The figure shows three views and two pictorial views of one solid part (mm, origin at its lowest corner). Answer the questions. Round coordinates to 2 decimals unless told otherwise and drop trailing zeros. Order: outer loops, then holes, each group sorted by start corner. A loop starts at its lowest first (then second) coordinate and runs counter-clockwise, first axis right, second up. Notation, with made-up numbers: (73, -40) - (95, -40) arc R16 cw to (95, -22) - close; hole circle Ø2 at (19.25, 76.5). An arc over 180 degrees is marked (long way). One line per question, with ' | ' between items. Start each with the question number.
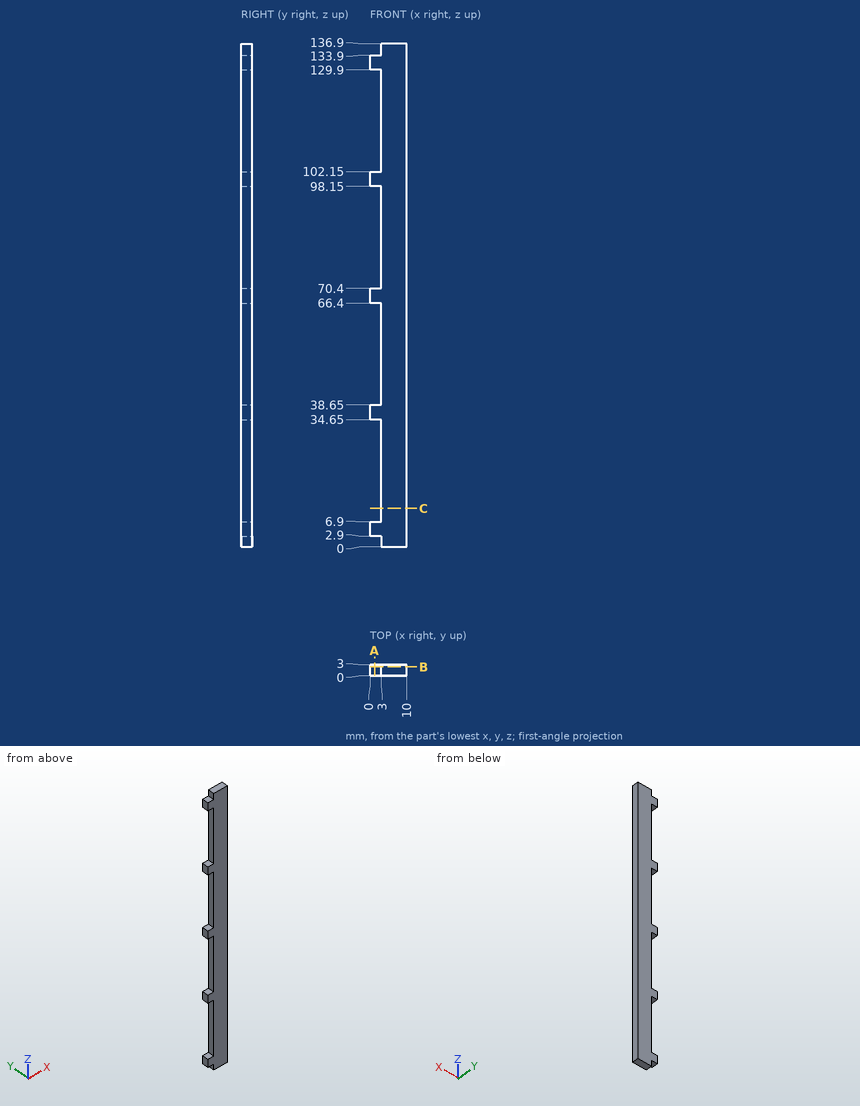
1) Flat-ended cylindrical pins translate along their axes: pin 1 (1.5 mm diameter, centred on x = 1.5, y = 1, fed in from -Z); pin 2 (1.5 mm diameter, centred on x = 1.5, y = 2, fed in from +Z); pin 3 (1.5 mm diameter, centred on y = 2, z = 57, fed in from -X). Find the tip coordinate at first contact, or state that the pin passes through.
2) Straight lines are drawn through the part: line 1 (Z direction, x = 1.25, y = 0.85); line 2 (X direction, y = 0.9, z = 9). For each, find the intervals that lie inside material, in ascending order.
3) Section B-B on y = 2.5 is taken. Give the vertices of the cut face in (x, z).
4) Section C-C on z = 10.5 is taken. Give the vertices of the cut face in (x, y), and give its area (3 significant figures).
5) Section A-A on x = 1.25 is taken. Give the vertices of the cut face in (y, z).
Recorded:
1) pin 1: stops at z = 2.9 | pin 2: stops at z = 133.9 | pin 3: stops at x = 3
2) line 1: z = 2.9 to 6.9, 34.65 to 38.65, 66.4 to 70.4, 98.15 to 102.15, 129.9 to 133.9 | line 2: x = 3 to 10
3) outline: (0, 2.9) - (3, 2.9) - (3, 0) - (10, 0) - (10, 136.9) - (3, 136.9) - (3, 133.9) - (0, 133.9) - (0, 129.9) - (3, 129.9) - (3, 102.15) - (0, 102.15) - (0, 98.15) - (3, 98.15) - (3, 70.4) - (0, 70.4) - (0, 66.4) - (3, 66.4) - (3, 38.65) - (0, 38.65) - (0, 34.65) - (3, 34.65) - (3, 6.9) - (0, 6.9) - close
4) outline: (3, 0) - (10, 0) - (10, 3) - (3, 3) - close | area: 21.0 mm²
5) outline: (0, 2.9) - (3, 2.9) - (3, 6.9) - (0, 6.9) - close; (0, 34.65) - (3, 34.65) - (3, 38.65) - (0, 38.65) - close; (0, 66.4) - (3, 66.4) - (3, 70.4) - (0, 70.4) - close; (0, 98.15) - (3, 98.15) - (3, 102.15) - (0, 102.15) - close; (0, 129.9) - (3, 129.9) - (3, 133.9) - (0, 133.9) - close
